Source: CAD feature listing. Evaluate the final solid. Frame: model axes, mm. A direction names the side the tool comes from. Give positions to 0.01 mm unless a question says otherwise; leave off trailing zeros. Write each loop counter-clockwise with the first axis right and the second up, starting at its lowest first coordinate (ties: lowest second). Pieces come first, ordered by that corner, then holes. Notation, with made-up numbers: (2, 34) -> (47, 34) arc R29 ccw to (47, 60) -> close; hole circle Ø7 at (56.25, 24). An arc over 180 degrees is marked (long way). Write item = value, one per line.
from build123d import *

# Parameters (mm, degrees)
F1_DEPTH  = 58
F2_R      = 2
F3_DEPTH  = 6.001
F4_R      = 7.5
F5_DEPTH  = 58.001
F7_DEPTH  = 43.001
F8_R      = 1.5
F9_DEPTH  = 2.4
F10_DEPTH = 5.001002


with BuildPart() as f1:
    # F0 (on Top) → F1 (new body)
    with BuildSketch(Plane.XY):
        Polygon((0, 67), (0, 0), (6, 0), (6, 72.000002), (-37, 72.000002), (-37, 67), align=None)
    extrude(amount=F1_DEPTH)

    # F2 (on face) → F3 (cut, through all)
    with BuildSketch(Plane(origin=(0, 0, 0), x_dir=(0, -1, 0), z_dir=(-1, 0, 0))):
        with Locations((-45, 37)):
            Circle(F2_R)
        with Locations((-45, 14)):
            Circle(F2_R)
        with Locations((-22, 14)):
            Circle(F2_R)
        with Locations((-22, 37)):
            Circle(F2_R)
    extrude(amount=-F3_DEPTH, mode=Mode.SUBTRACT)

    # F4 (on face) → F5 (cut, through all)
    with BuildSketch(Plane.XY):
        with Locations((-6, 11)):
            Circle(F4_R)
        with Locations((-6, 56)):
            Circle(F4_R)
    extrude(amount=F5_DEPTH, mode=Mode.SUBTRACT)

    # F6 (on face) → F7 (cut, through all)
    with BuildSketch(Plane.YZ.offset(6)):
        Polygon((60.000002, 51), (66.000002, 58), (0, 58), (0, 51), align=None)
    extrude(amount=-F7_DEPTH, mode=Mode.SUBTRACT)

    # F8 (on face) → F9 (cut)
    with BuildSketch(Plane.XZ.offset(-67)):
        Polygon((-7.75, 49.587713), (-7.75, 46.412287), (-5, 44.824574), (-2.25, 46.412287), (-2.25, 49.587713), (-5, 51.175426), align=None)
        with Locations((-5, 48)):
            Circle(F8_R, mode=Mode.SUBTRACT)
        Polygon((-2.25, 16.412287), (-2.25, 19.587713), (-5, 21.175426), (-7.75, 19.587713), (-7.75, 16.412287), (-5, 14.824574), align=None)
        with Locations((-5, 18)):
            Circle(F8_R, mode=Mode.SUBTRACT)
        Polygon((-11.25, 46.412287), (-11.25, 49.587713), (-14, 51.175426), (-16.75, 49.587713), (-16.75, 46.412287), (-14, 44.824574), align=None)
        with Locations((-14, 48)):
            Circle(F8_R, mode=Mode.SUBTRACT)
        Polygon((-11.25, 16.412287), (-11.25, 19.587713), (-14, 21.175426), (-16.75, 19.587713), (-16.75, 16.412287), (-14, 14.824574), align=None)
        with Locations((-14, 18)):
            Circle(F8_R, mode=Mode.SUBTRACT)
        Polygon((-20.25, 46.412287), (-20.25, 49.587713), (-23, 51.175426), (-25.75, 49.587713), (-25.75, 46.412287), (-23, 44.824574), align=None)
        with Locations((-23, 48)):
            Circle(F8_R, mode=Mode.SUBTRACT)
        Polygon((-20.25, 16.412287), (-20.25, 19.587713), (-23, 21.175426), (-25.75, 19.587713), (-25.75, 16.412287), (-23, 14.824574), align=None)
        with Locations((-23, 18)):
            Circle(F8_R, mode=Mode.SUBTRACT)
        Polygon((-29.25, 46.412287), (-29.25, 49.587713), (-32, 51.175426), (-34.75, 49.587713), (-34.75, 46.412287), (-32, 44.824574), align=None)
        with Locations((-32, 48)):
            Circle(F8_R, mode=Mode.SUBTRACT)
        Polygon((-29.25, 16.412287), (-29.25, 19.587713), (-32, 21.175426), (-34.75, 19.587713), (-34.75, 16.412287), (-32, 14.824574), align=None)
        with Locations((-32, 18)):
            Circle(F8_R, mode=Mode.SUBTRACT)
    extrude(amount=-F9_DEPTH, mode=Mode.SUBTRACT)

    # F8 (on face) → F10 (cut, through all)
    with BuildSketch(Plane.XZ.offset(-67)):
        with Locations((-32, 48)):
            Circle(F8_R)
        with Locations((-23, 48)):
            Circle(F8_R)
        with Locations((-14, 48)):
            Circle(F8_R)
        with Locations((-5, 48)):
            Circle(F8_R)
        with Locations((-32, 18)):
            Circle(F8_R)
        with Locations((-23, 18)):
            Circle(F8_R)
        with Locations((-14, 18)):
            Circle(F8_R)
        with Locations((-5, 18)):
            Circle(F8_R)
    extrude(amount=-F10_DEPTH, mode=Mode.SUBTRACT)


solid = f1.part
1) Cut plane D-D (z = 41). Return the cut outline in (x, y).
Computed:
outline = (-37, 67) -> (0, 67) -> (0, 60.5) arc R7.5 cw to (0, 51.5) -> (0, 15.5) arc R7.5 cw to (0, 6.5) -> (0, 0) -> (6, 0) -> (6, 72) -> (-37, 72) -> close
2) Cut plane C-C (z = 48). State how many separate pieces and enclosed holes the cut face has, then the cut area to 3 significant figures.
Computed:
separate_pieces = 5
enclosed_holes = 0
area = 515 mm²
3) Access query for faces 4 (the flat face through (-33.3, 69.4, 16.6)), 5 (the flat face through (-19, 67, 29)), 6 (the flat face through (0.3, 44.2, 0)). Directions: +Z, -Z, +X, -X, +Y, -Y. A direction counts if a zero-diameter tool reaches every point of the face in a straight line with its end or side. Return the directions, or none.
Computed:
face_4 = -Y
face_5 = +Z, -Z, -X, -Y
face_6 = -Z, +X, -X, +Y, -Y
4) Cut plane B-B (z = 14). Return the cut outline in (x, y), then the cut area to 3 significant figures.
Computed:
outline = (-37, 67) -> (0, 67) -> (0, 60.5) arc R7.5 cw to (0, 51.5) -> (0, 47) -> (6, 47) -> (6, 72) -> (-37, 72) -> close; (0, 0) -> (6, 0) -> (6, 20) -> (0, 20) -> (0, 15.5) arc R7.5 cw to (0, 6.5) -> close; (0, 24) -> (6, 24) -> (6, 43) -> (0, 43) -> close
area = 551 mm²
5) Contact query for flat-ended pins moving along their axis: pin 1 (3 mm diameter, centred on x = -5.5, z = 46.5, fed in from -Y); pin 2 (2 mm diameter, centred on y = 4, z = 34, fed in from -X); pin 3 (6.5 mm diameter, centred on x = 2, y = 27.5, fed in from +Z); pin 4 (4 mm diameter, centred on x = -14, z = 18, fed in from +Y). Output: stop coordinate, or through.
Computed:
pin_1 = 67
pin_2 = 0
pin_3 = 51
pin_4 = 72
6) Material intervals for L1, parallel to Z at x = 4.7, y = 45; L2, parallel to Z at x = -32, y = 71.45; L3, parallel to Y at x = -11, z = 28, sorted ascending.
Computed:
L1 = 0 to 12, 16 to 35, 39 to 51
L2 = 0 to 16.5, 19.5 to 46.5, 49.5 to 58
L3 = 67 to 72
7) Draft query along X for faces 1 (the flat face through (-30.64, 68.18, 15.61)), 2 (the cylindrical face through (3, 22, 35)), 3 (the flat face through (0, 64, 29)). Return one class per face: pulls with the +X half, pulls with the -X half, needs draft (parallel to the pull), parting line crosses it, or undercut.
Computed:
face_1 = undercut
face_2 = needs draft
face_3 = pulls with the -X half
8) Cut plane A-A (y = 45). Return the cut outline in (x, z), then the cut area to 3 significant figures.
Computed:
outline = (0, 0) -> (6, 0) -> (6, 12) -> (0, 12) -> close; (0, 16) -> (6, 16) -> (6, 35) -> (0, 35) -> close; (0, 39) -> (6, 39) -> (6, 51) -> (0, 51) -> close
area = 258 mm²
